Input: part model. Units: mm. Frame: model coordinates. A direction names the side the tool comes from. Coordinates: 2 decimals unless noted, no trailing zeros. Order: outer loops, then holes, each group sorted by start corner. A loop starts at its lowest first (then second) coordinate and runs counter-clockwise, first axis right, second up. Notation, with made-up numbers: M -28.75,66.25 L -0.75,66.25 A18 cw -0.75,100.25 Z; hole C -1,-10 d8. An arc over 180 degrees is marked long. One line per item, written item: value.
Autodesk Fusion 360 part; units mm, degrees
sketch "Sketch1" plane through (0, 0, 0) normal (0, 1, 0) x (1, 0, 0)
  line L0 (-20, 10) -> (3, 10)
  line L1 (3, 10) -> (3, -2.3)
  line L2 (3, -2.3) -> (-20, -2.3)
  line L3 (-20, -2.3) -> (-20, 10)
  dimension "d1" = 23
  dimension "d2" = 12.3
extrude "Extrude1" add sketch "Sketch1" along normal blind 15.4 makes body 1
sketch "Sketch2" plane through (0, 15.4, 0) normal (0, 1, 0) x (-1, 0, 0)
  line L0 (20, 2.3) -> (-3, 2.3)
  line L1 (-3, 2.3) -> (-3, -10)
  line L2 (-3, -10) -> (20, -10)
  line L3 (20, -10) -> (20, 2.3)
  line L4 (24.6, -10) -> (-7.6, -10)
  line L5 (-7.6, -10) -> (-7.6, 2.3)
  line L6 (-7.6, 2.3) -> (24.6, 2.3)
  line L7 (24.6, 2.3) -> (24.6, -10)
  line L8 (24.6, -10) -> (-7.6, 2.3) construction
  line L9 (-7.6, -10) -> (24.6, 2.3) construction
  line L10 (20, -3.85) -> (24.6, -3.85) construction
  line L11 (-3, -3.85) -> (-7.6, -3.85) construction
  circle A0 centre (-5.3, -3.85) radius 1
  circle A1 centre (22.3, -3.85) radius 1
  point P0 (8.5, -3.85)
  dimension "d5" = 32.2
  dimension "d6" = 2
  dimension "d7" = 2
extrude "Extrude2" add sketch "Sketch2" along normal blind 2.5 bodies 1
sketch "Sketch3" plane through (0, 17.9, 0) normal (0, 1, 0) x (-1, 0, 0)
  circle A0 centre (-5.3, -3.85) radius 1
  circle A1 centre (22.3, -3.85) radius 1
  line L0 (24.6, 2.3) -> (-7.6, 2.3)
  line L1 (-7.6, 2.3) -> (-7.6, -10)
  line L2 (-7.6, -10) -> (24.6, -10)
  line L3 (24.6, -10) -> (24.6, 2.3)
  line L4 (-3, 2.3) -> (20, 2.3)
  line L5 (20, 2.3) -> (20, -10)
  line L6 (20, -10) -> (-3, -10)
  line L7 (-3, -10) -> (-3, 2.3)
extrude "Extrude3" add sketch "Sketch3" along normal blind 4.2 contours L0 L2 L4 L5 L6 L7 bodies 1
sketch "Sketch4" plane through (0, 22.1, 0) normal (0, 1, 0) x (-1, 0, 0)
  line L0 (-3, -10) -> (20, -10)
  line L1 (20, -10) -> (20, 2.3)
  line L2 (20, 2.3) -> (-3, 2.3)
  line L3 (-3, 2.3) -> (-3, -10)
  circle A0 centre (13.85, -3.85) radius 6.15
  circle A1 centre (7, -4) radius 2.8
  line L4 (12.5, -6.8) -> (1.5, -6.8)
  line L5 (1.5, -6.8) -> (1.5, -1.2)
  line L6 (1.5, -1.2) -> (12.5, -1.2)
  line L7 (12.5, -1.2) -> (12.5, -6.8)
  line L8 (12.5, -6.8) -> (1.5, -1.2) construction
  line L9 (1.5, -6.8) -> (12.5, -1.2) construction
  point P0 (7, -4)
  dimension "d12" = 5.6
  dimension "d13" = 5.6
extrude "Extrude4" add sketch "Sketch4" along normal blind 4.3 contours A0 L4 L6 L7 | A0 A1 L4 | A0 A1 L4 L6 L7 | A0 A1 | A0 A1 | A0 A1 L6 bodies 1
sketch "Sketch5" plane through (0, 26.4, 0) normal (0, 1, 0) x (-1, 0, 0)
  arc A0 (7, -1.2) -> (7, -6.8) centre (7, -4) ccw
  line L0 (7, -6.8) -> (8.4537, -6.8)
  arc A1 (8.4537, -6.8) -> (8.3002, -1.2) centre (13.85, -3.85) ccw
  line L1 (8.3002, -1.2) -> (7, -1.2)
  circle A2 centre (13.85, -3.85) radius 3.5
  dimension "d16" = 7
extrude "Extrude5" add sketch "Sketch5" along normal blind 5 contours A2 bodies 1
sketch "Sketch6" plane through (0, 31.4, 0) normal (0, 1, 0) x (-1, 0, 0)
  circle A0 centre (13.85, -3.85) radius 3.5
  line L0 (13.85, -3.85) -> (28.85, -3.85)
  circle A1 centre (28.85, -3.85) radius 2
  line L1 (15.7335, -6.8) -> (15.7335, -0.9)
  line L2 (15.7335, -6.8) -> (28.9937, -5.8448)
  line L3 (15.7335, -0.9) -> (28.9937, -1.8552)
  dimension "d19" = 15
  dimension "d20" = 4
  dimension "d21" = 5.9
extrude "Extrude6" add sketch "Sketch6" against normal blind 1.4 contours A0 L0 A1 L2 | A0 L0 A1 L3 | A1 bodies 1
sketch "Sketch7" plane through (0, 31.4, 0) normal (0, 1, 0) x (-1, 0, 0)
  arc A0 (15.7335, -0.9) -> (15.7335, -6.8) centre (13.85, -3.85) ccw
  line L0 (15.7335, -6.8) -> (28.9937, -5.8448)
  arc A1 (28.9937, -5.8448) -> (28.9937, -1.8552) centre (28.85, -3.85) ccw
  line L1 (28.9937, -1.8552) -> (15.7335, -0.9)
  circle A2 centre (13.85, -3.85) radius 3.5 construction
  circle A3 centre (28.85, -3.85) radius 0.5
  line L2 (17.35, -3.85) -> (28.85, -3.85) construction
  circle A4 centre (26.9333, -3.85) radius 0.5
  circle A5 centre (25.0167, -3.85) radius 0.5
  circle A6 centre (23.1, -3.85) radius 0.5
  circle A7 centre (21.1833, -3.85) radius 0.5
  circle A8 centre (19.2667, -3.85) radius 0.5
  circle A9 centre (17.35, -3.85) radius 0.5
  dimension "d24" = 1
  dimension "d27" = -11.5
  dimension "d28" = 0
extrude "Extrude7" cut sketch "Sketch7" against normal up to surface (1.4 mm away) contours A3 | A4 | A5 | A6 | A7 | A8 bodies 1
sketch "Sketch8" plane through (0, 31.4, 0) normal (0, 1, 0) x (-1, 0, 0)
  circle A0 centre (25.0167, -3.85) radius 0.5
  circle A1 centre (19.2667, -3.85) radius 0.5
  circle A2 centre (26.9333, -3.85) radius 0.5
  circle A3 centre (23.1, -3.85) radius 0.5
  circle A4 centre (21.1833, -3.85) radius 0.5
  circle A5 centre (28.85, -3.85) radius 0.5
  arc A6 (15.7335, -0.9) -> (15.7335, -6.8) centre (13.85, -3.85) ccw
  line L0 (15.7335, -6.8) -> (28.9937, -5.8448)
  arc A7 (28.9937, -5.8448) -> (28.9937, -1.8552) centre (28.85, -3.85) ccw
  line L1 (28.9937, -1.8552) -> (15.7335, -0.9)
  circle A8 centre (13.85, -3.85) radius 2.3
  dimension "d31" = 4.6
extrude "Extrude8" cut sketch "Sketch8" against normal blind 1 contours A8 bodies 1
sketch "Sketch9" plane through (0, 30.4, 0) normal (0, 1, 0) x (-1, 0, 0)
  circle A0 centre (13.85, -3.85) radius 2.3
  circle A1 centre (13.85, -3.85) radius 1.2
  dimension "d34" = 2.4
extrude "Extrude9" cut sketch "Sketch9" against normal blind 3 contours A1 bodies 1
copy_body "Body->Comp1" bodies 1 removing the originals makes body 2 in component "Servo"
component "Servo" placed x (1, 0, 0) y (0, 1, 0) z (0, 0, 1) at (0, 0, 0)
(1) Ray query, line 1 (Z direction, x = -22.3, y = 17.3); line 2 (Y direction, x = -19, z = -5.25); line 3 (X direction, y = 11, z = -1.75). Return the intervals inside material, ascending. Write a range as from..to.
Data:
line 1: z = -10..-4.85, -2.85..2.3
line 2: y = 0..26.4, 30..31.4
line 3: x = -20..3
(2) Draft query along X for faces 4 (the cylindrical face through (-10.353, 28.865, -4.004)), 5 (the cylindrical face through (-29.327, 30.71, -3.7)), 6 (the cylindrical face through (-30.85, 30.71, -3.89)). Return one class per face: released by +X, released by -X, zero draft, split by the parting line, or undercut.
Data:
face 4: split by the parting line
face 5: undercut
face 6: released by -X
(3) Cut plane A-A on z = -8.5. Output: boundary loops of the cut face in (x, y), plus the area to 3 significant figures.
Data:
outline: M -24.6,15.4 L -20,15.4 L -20,0 L 3,0 L 3,15.4 L 7.6,15.4 L 7.6,17.9 L 3,17.9 L 3,22.1 L -9.83,22.1 L -9.83,26.4 L -17.87,26.4 L -17.87,22.1 L -20,22.1 L -20,17.9 L -24.6,17.9 Z
area: 566 mm2
(4) Access query for faces 1 (the flat face through (-24.6, 17, -4)), 2 (the flat face through (5, 15.4, -5)), 3 (the flat face through (-10, 26.4, -4)). Directions: +Z, -Z, +X, -X, +Y, -Y. A direction counts if a zero-diameter tool reaches every point of the face in a straight line with its end or side. Return the directions, or none.
Data:
face 1: +Z, -Z, -X, -Y
face 2: +Z, -Z, +X, -Y
face 3: none
(5) Cut plane C-C on x = -12. Output: boundary loops of the cut face in (y, z), plus the area to 3 significant figures.
Data:
outline: M 0,-10 L 22.1,-10 L 22.1,-9.72 L 26.4,-9.72 L 26.4,-6.82 L 31.4,-6.82 L 31.4,-5.22 L 30.4,-5.22 L 30.4,-2.48 L 31.4,-2.48 L 31.4,-0.88 L 26.4,-0.88 L 26.4,2.02 L 22.1,2.02 L 22.1,2.3 L 0,2.3 Z
area: 349 mm2
(6) Cut plane D-D on y = 4.5. Output: boundary loops of the cut face in (x, z), plus the area to 3 significant figures.
Data:
outline: M -20,-10 L 3,-10 L 3,2.3 L -20,2.3 Z
area: 283 mm2
(7) First-contact query: pin 1 (3 mm diameter, centred on x = -6.5, z = -5.5, fed in from +Y); pin 2 (1.4 mm diameter, centred on x = -7.5, y = 25, fed in from +Z); pin 3 (1.4 mm diameter, centred on x = 5, z = -6, fed in from +Y). Flat tips, straight axial feed; report the tip coordinate or a pass-through.
Data:
pin 1: stops at y = 26.4
pin 2: stops at z = -1.2
pin 3: stops at y = 17.9
(8) Cut plane B-B on y = 23.5. Output: boundary loops of the cut face in (x, z), plus the area to 3 significant figures.
Data:
outline: M -8.45,-6.8 L -7,-6.8 A2.8 ccw -7,-1.2 L -8.3,-1.2 A6.15 ccw long Z
area: 136 mm2
